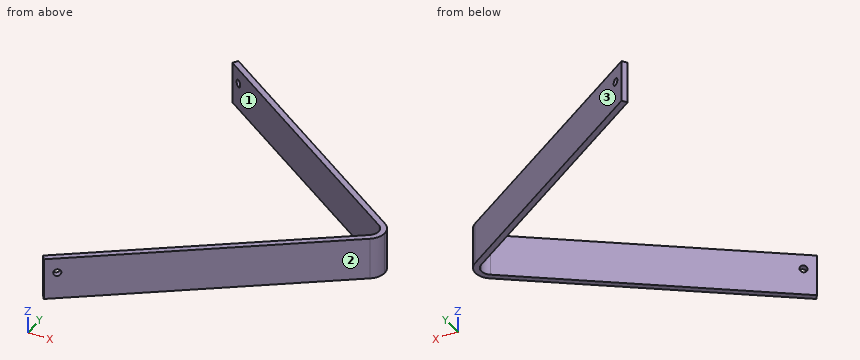
from build123d import *

# Parameters (mm, degrees)
PAD002_DEPTH           = 70
SKETCH006_R            = 6
POCKET002_DEPTH        = 30
SKETCH007_R            = 6
POCKET003_DEPTH        = 243.806754
LINEARPATTERN001_COUNT = 4
LINEARPATTERN001_PITCH = 140


with BuildPart() as part:
    # Sketch004 → Pad002 (new body)
    with BuildSketch(Plane.XY):
        with BuildLine():
            Line((-379.627892, 300), (16.06014, 22.936257))
            ThreePointArc((28, 0), (24.836303, 12.928961), (16.06014, 22.936257))
            Line((18, 0), (28, 0))
            ThreePointArc((18, 0), (15.966195, 8.311475), (10.324376, 14.744737))
            Line((10.324376, 14.744737), (-385.363656, 291.80848))
            Line((-385.363656, 291.80848), (-379.627892, 300))
        make_face()
    extrude(amount=PAD002_DEPTH)

    # Sketch006 → Pocket002 (cut)
    with BuildSketch(Plane(origin=(0, 126.75, 0), x_dir=(-1, 0, 0), z_dir=(0, 1, 0))):
        with Locations((26.740569, 25.24131)):
            Circle(SKETCH006_R)
    extrude(amount=-POCKET002_DEPTH, mode=Mode.SUBTRACT)

    # Sketch007 (on Face2 of Pocket002) → Pocket003 (cut, through all)
    with BuildSketch(Plane(origin=(10.324376, 14.744737, 0), x_dir=(0.819152, -0.573576, 0), z_dir=(-0.573576, -0.819152, 0))):
        with Locations((-463.045894, 45)):
            Circle(SKETCH007_R)
    pocket003 = extrude(amount=-POCKET003_DEPTH, mode=Mode.SUBTRACT)

    # LinearPattern001: Pocket003 ×4
    with Locations(*[Vector(-0.819152, 0.573576, 0) * (i * LINEARPATTERN001_PITCH) for i in range(1, LINEARPATTERN001_COUNT)]):
        add(pocket003, mode=Mode.SUBTRACT)

    # Mirrored001: part across XZ


with BuildPart() as part_1:
    add(part.part)
    add(part.part.mirror(Plane.XZ))


with BuildPart() as part_2:
    # Body001 placement: moved
    add(part_1.part.moved(Location((0, 0, -20))))


solid = part_2.part
Input: part model. Units: mm. Frame: model coordinates. Face numbers are marked on the shaded views. Round coordinates to 2 decimals unless told otherwise and drop trailing zeros. Order: outer loops, then holes, each group sorted by start corner. A loop starts at its lowest first (then second) coordinate and runs counter-clockwise, first axis right, second up.
1. Material intervals for line 1 (Y direction, x = 2, z = 45); line 2 (Y direction, x = -45.5, z = -11.5); line 3 (X direction, y = 161.5, z = 24.5), sorted ascending.
The answers:
line 1: y = -32.78 to -20.57, 20.57 to 32.78
line 2: y = -66.04 to -53.83, 53.83 to 66.04
line 3: x = -199.26 to -181.83
2. Pin query (flat end, axial travel): P1, Ø1.5, axis at y = 177.5, z = 2, coming from the +X side; P2, Ø1.5, axis at x = -280.5, z = 36.5, coming from the -Y side; P3, Ø2, axis at x = -31.5, z = 19, coming from the +Y side. Return the tip coordinate at first contact, or that it passes through.
The answers:
P1: stops at x = -203.61
P2: stops at y = -231.12
P3: stops at y = 56.94
3. Mould query, pull axis Y, two halves, no side actions, for the marked faces 1, 2 and 3. Classes: released by +Y, released by -Y, zero draft, split by the parting line, or undercut.
The answers:
face 1: undercut
face 2: released by -Y
face 3: released by +Y
4. Cut plane C-C, the plane y = -8. Output: boundary loops of the cut face in (x, z), then the cut area to 3 significant figures.
The answers:
outline: (16.12, -20) - (26.83, -20) - (26.83, 50) - (16.12, 50) - close
area: 750 mm2
5. Cut plane B-B, the plane x = -331.5. Output: boundary loops of the cut face in (y, z), then the cut area to 3 significant figures.
The answers:
outline: (-266.3, -20) - (-254.09, -20) - (-254.09, 50) - (-266.3, 50) - close; (254.09, -20) - (266.3, -20) - (266.3, 50) - (254.09, 50) - close
area: 1,710 mm2
6. Cut plane A-A, the plane z = 1. Output: boundary loops of the cut face in (x, y), then the cut area to 3 significant figures.
The answers:
outline: (-385.36, -291.81) - (-379.63, -300) - (16.06, -22.94) arc R28 ccw to (28, 0) arc R28 ccw to (16.06, 22.94) - (-379.63, 300) - (-385.36, 291.81) - (10.32, 14.74) arc R18 cw to (10.32, -14.74) - close
area: 10,100 mm2
7. Cut plane D-D, the plane y = -96. Output: boundary loops of the cut face in (x, z), then the cut area to 3 significant figures.
The answers:
outline: (-105.72, -20) - (-88.29, -20) - (-88.29, 50) - (-105.72, 50) - close
area: 1,220 mm2
